Source: three-view drawing plus pictorial views. Frame: mm from the lowest corner of the part. A direction names the side the tool comes from. Give positions to 0.01 mm unless a question says otherwise; leave off trailing zeros. Loops run counter-clockwise (first coordinate to the right, second up) from the corner with the lowest first, then second, coordinate; pieces in that order, holes last.
1. Draft query along X for the marked faces 1, 2, 3 and 4. Return one class per face: +X half, -X half, draft (parallel to the pull), parting line (faces both ways), or undercut.
2. Material intervals for line 1 along X through (y, z) = (70, 5); line 2 along Y through (x, z) = (37.5, 9.75); line 3 along Z through (x, y) = (15, 52), sorted ascending.
3. Section C-C, the plane z = 7.25. Output: boundary loops of the cut face in (x, y) (3 decimals).
4. Section A-A, the plane y = 20. Output: boundary loops of the cut face in (x, z), then the cut area to 3 significant figures.
5. Section B-B, the plane x = 40.5. Output: boundary loops of the cut face in (y, z), then the cut area to 3 significant figures.
6. Access query for the marked faces 5 and 6. Directions: +Z, -Z, +X, -X, +Y, -Y. A direction counts if a zero-diameter tool reaches every point of the face in a straight line with its end or side. Return the directions, or none.
7. First-contact query: P1, Ø3, axis at x = 5.5, y = 62.5, coming from the -Z side; P2, Ø10, axis at x = 42.5, y = 17, coming from the +Z side; P3, Ø3, axis at x = 26, z = 9.5, coming from the -Y side. Flat tips, straight axial feed; report the tip coordinate or a pass-through.
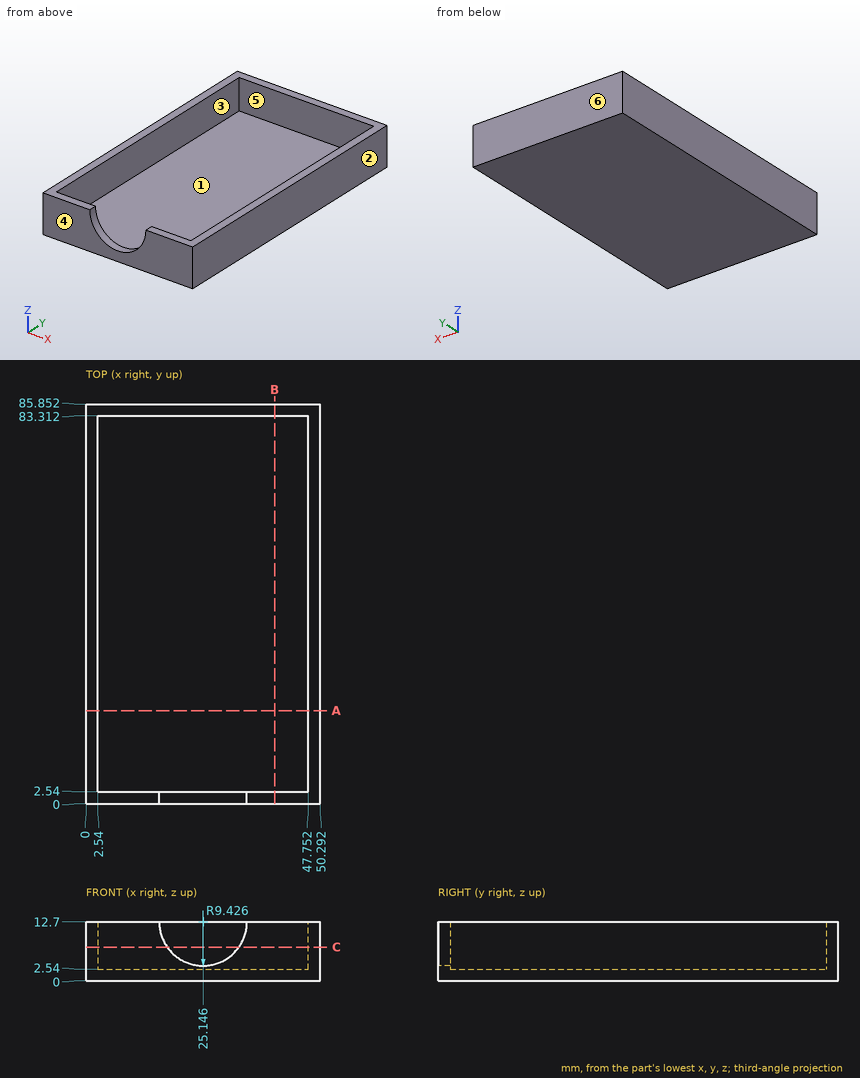
Answers below:
1. face 1: undercut
1. face 2: +X half
1. face 3: undercut
1. face 4: draft
2. line 1: x = 0 to 2.54, 47.75 to 50.29
2. line 2: y = 0 to 2.54, 83.31 to 85.85
2. line 3: z = 0 to 2.54
3. outline: (0, 0) - (17.455, 0) - (17.455, 2.54) - (2.54, 2.54) - (2.54, 83.312) - (47.752, 83.312) - (47.752, 2.54) - (32.837, 2.54) - (32.837, 0) - (50.292, 0) - (50.292, 85.852) - (0, 85.852) - close
4. outline: (0, 0) - (50.29, 0) - (50.29, 12.7) - (47.75, 12.7) - (47.75, 2.54) - (2.54, 2.54) - (2.54, 12.7) - (0, 12.7) - close
4. area: 179 mm2
5. outline: (0, 0) - (85.85, 0) - (85.85, 12.7) - (83.31, 12.7) - (83.31, 2.54) - (2.54, 2.54) - (2.54, 12.7) - (0, 12.7) - close
5. area: 270 mm2
6. face 5: +Z
6. face 6: +Z, -Z, +X, -X, +Y
7. P1: stops at z = 0
7. P2: stops at z = 2.54
7. P3: stops at y = 83.31
